Study the drawing (mm; zero at the part's minimum x, y, z) and answer. A direction names the side the tool comes from. Coordinates: 2 decimals unless noted, no trailing zeros. Write each loop counter-clockwise with the first axis right and the second up, starting at its lowest first coordinate (ties: lowest second). Pieces come first, ordered by that corner, then holes. Notation, with made-up numbers: (82.5, 10.25) -> (93.5, 10.25) arc R5 cw to (93.5, 18.25) -> close; hole circle Ø4 at (-32, 78.5). An arc over 180 degrees is marked (long way). Answer in a Markdown table with one row per item. Add a question column.
Item 1: Section D-D on y = 2.75 is taken. Write down the section's boundary in (x, z), then the cut area to 3 significant figures.
Item 2: Given pin 1 Ø3 at (y, z) = (3.5, 9) entering from -X; pin 2 Ø1.6 at (y, z) = (6.5, 9.5) entering from +X; pin 3 Ø4 at (y, z) = (2, 7) entering from -X, each flat-ended and moving along its own axis, determine where each tip first touches the part or whether it passes through.
Item 3: For a pull along Z with two mould halves and no side action, classify the marked faces 4, 5 and 6 as +Z half, -Z half, draft (parallel to the pull), parting line (faces both ways), or undercut.
Item 4: Section A-A on x = 6 is taken. Write down the section's boundary in (y, z).
Item 5: Section C-C on z = 8.25 is taken. Write down the section's boundary in (x, y) (1 decimal).
Item 6: Which of the six approach directions +Z, -Z, +X, -X, +Y, -Y give full straight-line access (tool end or side, diameter ignored) to the marked faces 1, 2 and 3?
Item 7: Straight lines are drawn through the part: line 1 (Z direction, x = 6, y = 5.25); line 2 (X direction, y = 6.75, z = 13.25); line 3 (Z direction, x = 7.75, y = 5.5) (1 decimal). For each, find the intervals that lie inside material, in ascending order. Write a range as from..to.
Item 8: Section B-B on z = 10.75 is taken. Write down the section's boundary in (x, y) (1 decimal).
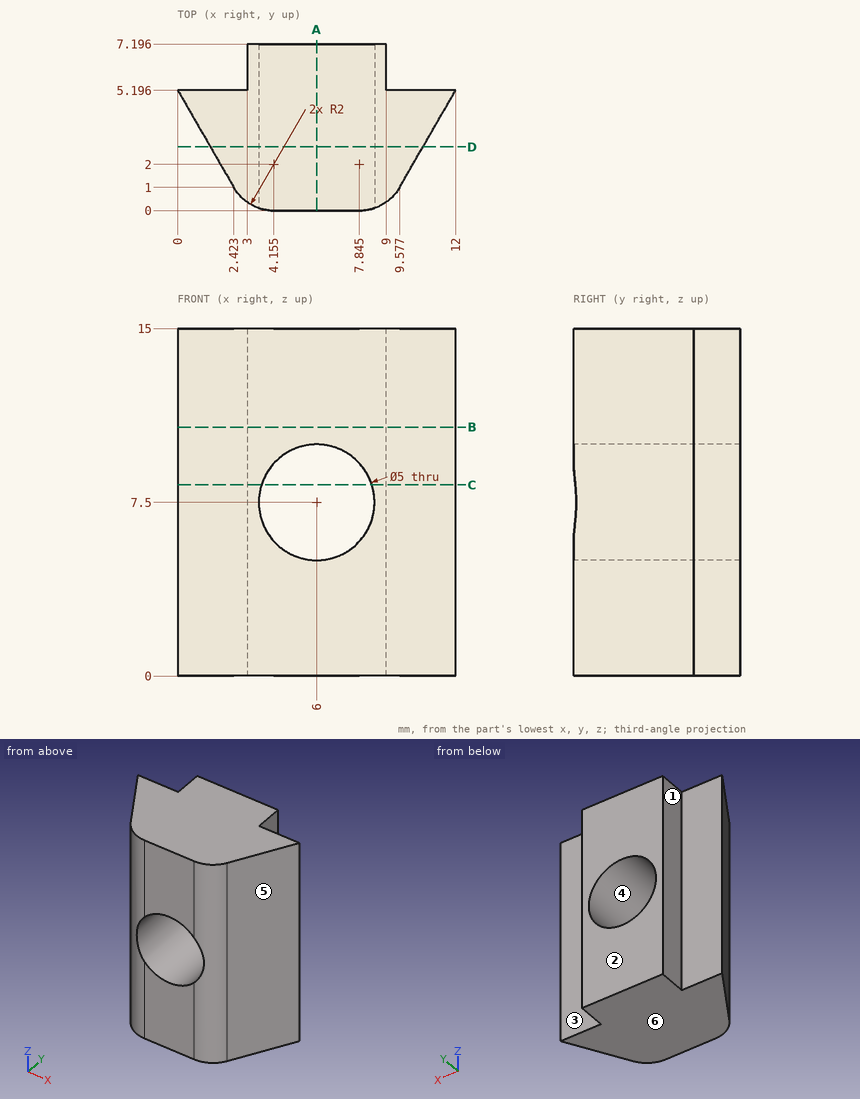
Results below:
| question | item | result |
|---|---|---|
| 1 | outline | (1.41, 0) -> (10.59, 0) -> (10.59, 15) -> (1.41, 15) -> close; hole circle Ø5 at (6, 7.5) |
| 1 | area | 118 mm2 |
| 2 | pin 1 | stops at x = 0.11 |
| 2 | pin 2 | stops at x = 9 |
| 2 | pin 3 | stops at x = 0.69 |
| 3 | face 4 | undercut |
| 3 | face 5 | draft |
| 3 | face 6 | -Z half |
| 4 | outline | (0, 0) -> (7.2, 0) -> (7.2, 5) -> (0, 5) -> close; (0, 10) -> (7.2, 10) -> (7.2, 15) -> (0, 15) -> close |
| 5 | outline | (0, 5.2) -> (2.4, 1) arc R2 ccw to (3.6, 0.1) -> (3.6, 7.2) -> (3, 7.2) -> (3, 5.2) -> close; (8.4, 0.1) arc R2 ccw to (9.6, 1) -> (12, 5.2) -> (9, 5.2) -> (9, 7.2) -> (8.4, 7.2) -> close |
| 6 | face 1 | +Z, -Z, -X, +Y |
| 6 | face 2 | +Z, -Z, +X, -X, +Y |
| 6 | face 3 | +Z, -Z, +X, +Y |
| 7 | line 1 | z = 0..5, 10..15 |
| 7 | line 2 | x = 3..9 |
| 7 | line 3 | z = 0..5.7, 9.3..15 |
| 8 | outline | (0, 5.2) -> (2.4, 1) arc R2 ccw to (4.2, 0) -> (7.8, 0) arc R2 ccw to (9.6, 1) -> (12, 5.2) -> (9, 5.2) -> (9, 7.2) -> (3, 7.2) -> (3, 5.2) -> close |
